```python
from build123d import *

# Parameters (mm, degrees)
SKETCH1_W                = 100
SKETCH1_H                = 67.6
BOSS_EXTRUDE1_DEPTH      = 3
SKETCH3_W                = 4
SKETCH3_H                = 3
CUT_EXTRUDE1_DEPTH       = 10
LPATTERN1_COUNT          = 13
LPATTERN1_PITCH          = 8
SKETCH7_W                = 15
SKETCH7_H                = 45
CUT_EXTRUDE5_DEPTH       = 3
MIRROR1_COPY_1_SKETCH_W  = 4
MIRROR1_COPY_1_SKETCH_H  = 3
MIRROR1_COPY_1_DEPTH     = 10
MIRROR1_COPY_2_SKETCH_W  = 4
MIRROR1_COPY_2_SKETCH_H  = 3
MIRROR1_COPY_2_DEPTH     = 10
MIRROR1_COPY_3_SKETCH_W  = 4
MIRROR1_COPY_3_SKETCH_H  = 3
MIRROR1_COPY_3_DEPTH     = 10
MIRROR1_COPY_4_SKETCH_W  = 4
MIRROR1_COPY_4_SKETCH_H  = 3
MIRROR1_COPY_4_DEPTH     = 10
MIRROR1_COPY_5_SKETCH_W  = 4
MIRROR1_COPY_5_SKETCH_H  = 3
MIRROR1_COPY_5_DEPTH     = 10
MIRROR1_COPY_6_SKETCH_W  = 4
MIRROR1_COPY_6_SKETCH_H  = 3
MIRROR1_COPY_6_DEPTH     = 10
MIRROR1_COPY_7_SKETCH_W  = 4
MIRROR1_COPY_7_SKETCH_H  = 3
MIRROR1_COPY_7_DEPTH     = 10
MIRROR1_COPY_8_SKETCH_W  = 4
MIRROR1_COPY_8_SKETCH_H  = 3
MIRROR1_COPY_8_DEPTH     = 10
MIRROR1_COPY_9_SKETCH_W  = 4
MIRROR1_COPY_9_SKETCH_H  = 3
MIRROR1_COPY_9_DEPTH     = 10
MIRROR1_COPY_10_SKETCH_W = 4
MIRROR1_COPY_10_SKETCH_H = 3
MIRROR1_COPY_10_DEPTH    = 10
MIRROR1_COPY_11_SKETCH_W = 4
MIRROR1_COPY_11_SKETCH_H = 3
MIRROR1_COPY_11_DEPTH    = 10
MIRROR1_COPY_12_SKETCH_W = 4
MIRROR1_COPY_12_SKETCH_H = 3
MIRROR1_COPY_12_DEPTH    = 10
LPATTERN2_COUNT          = 2
LPATTERN2_PITCH          = 30
LPATTERN2_COL_COUNT      = 2
LPATTERN2_COL_PITCH      = 30
SKETCH8_W                = 4
SKETCH8_H                = 8.2
SKETCH8_H_2              = 33.8
BOSS_EXTRUDE2_DEPTH      = 3
CUT_EXTRUDE6_REACH       = 5
SKETCH9_W                = 12
SKETCH9_H                = 3


with BuildPart() as part:
    # Sketch1 → Boss-Extrude1 (new body)
    with BuildSketch(Plane.XY):
        Rectangle(SKETCH1_W, SKETCH1_H)
    extrude(amount=BOSS_EXTRUDE1_DEPTH)

    # Sketch3 → Cut-Extrude1 (cut)
    with BuildSketch(Plane(origin=(0, 0, 0), x_dir=(-1, 0, 0), z_dir=(0, 0, -1))):
        with Locations((-48, -32.3)):
            Rectangle(SKETCH3_W, SKETCH3_H)
    cut_extrude1 = extrude(amount=-CUT_EXTRUDE1_DEPTH, mode=Mode.SUBTRACT)

    # LPattern1: Cut-Extrude1 ×13
    with Locations(*[(-i * LPATTERN1_PITCH, 0, 0) for i in range(1, LPATTERN1_COUNT)]):
        add(cut_extrude1, mode=Mode.SUBTRACT)

    # Sketch7 → Cut-Extrude5 (cut)
    with BuildSketch(Plane(origin=(0, 0, 0), x_dir=(-1, 0, 0), z_dir=(0, 0, -1))):
        Rectangle(SKETCH7_W, SKETCH7_H)
    cut_extrude5 = extrude(amount=-CUT_EXTRUDE5_DEPTH, mode=Mode.SUBTRACT)

    # Mirror1: Cut-Extrude1 across plane
    add(cut_extrude1.mirror(Plane.ZX), mode=Mode.SUBTRACT)

    # Mirror1 copy 1 sketch → Mirror1 copy 1 (cut)
    with BuildSketch(Plane(origin=(-8, 0, 0), x_dir=(-1, 0, 0), z_dir=(0, 0, -1))):
        with Locations((-48, 32.3)):
            Rectangle(MIRROR1_COPY_1_SKETCH_W, MIRROR1_COPY_1_SKETCH_H)
    extrude(amount=-MIRROR1_COPY_1_DEPTH, mode=Mode.SUBTRACT)

    # Mirror1 copy 2 sketch → Mirror1 copy 2 (cut)
    with BuildSketch(Plane(origin=(-16, 0, 0), x_dir=(-1, 0, 0), z_dir=(0, 0, -1))):
        with Locations((-48, 32.3)):
            Rectangle(MIRROR1_COPY_2_SKETCH_W, MIRROR1_COPY_2_SKETCH_H)
    extrude(amount=-MIRROR1_COPY_2_DEPTH, mode=Mode.SUBTRACT)

    # Mirror1 copy 3 sketch → Mirror1 copy 3 (cut)
    with BuildSketch(Plane(origin=(-24, 0, 0), x_dir=(-1, 0, 0), z_dir=(0, 0, -1))):
        with Locations((-48, 32.3)):
            Rectangle(MIRROR1_COPY_3_SKETCH_W, MIRROR1_COPY_3_SKETCH_H)
    extrude(amount=-MIRROR1_COPY_3_DEPTH, mode=Mode.SUBTRACT)

    # Mirror1 copy 4 sketch → Mirror1 copy 4 (cut)
    with BuildSketch(Plane(origin=(-32, 0, 0), x_dir=(-1, 0, 0), z_dir=(0, 0, -1))):
        with Locations((-48, 32.3)):
            Rectangle(MIRROR1_COPY_4_SKETCH_W, MIRROR1_COPY_4_SKETCH_H)
    extrude(amount=-MIRROR1_COPY_4_DEPTH, mode=Mode.SUBTRACT)

    # Mirror1 copy 5 sketch → Mirror1 copy 5 (cut)
    with BuildSketch(Plane(origin=(-40, 0, 0), x_dir=(-1, 0, 0), z_dir=(0, 0, -1))):
        with Locations((-48, 32.3)):
            Rectangle(MIRROR1_COPY_5_SKETCH_W, MIRROR1_COPY_5_SKETCH_H)
    extrude(amount=-MIRROR1_COPY_5_DEPTH, mode=Mode.SUBTRACT)

    # Mirror1 copy 6 sketch → Mirror1 copy 6 (cut)
    with BuildSketch(Plane(origin=(-48, 0, 0), x_dir=(-1, 0, 0), z_dir=(0, 0, -1))):
        with Locations((-48, 32.3)):
            Rectangle(MIRROR1_COPY_6_SKETCH_W, MIRROR1_COPY_6_SKETCH_H)
    extrude(amount=-MIRROR1_COPY_6_DEPTH, mode=Mode.SUBTRACT)

    # Mirror1 copy 7 sketch → Mirror1 copy 7 (cut)
    with BuildSketch(Plane(origin=(-56, 0, 0), x_dir=(-1, 0, 0), z_dir=(0, 0, -1))):
        with Locations((-48, 32.3)):
            Rectangle(MIRROR1_COPY_7_SKETCH_W, MIRROR1_COPY_7_SKETCH_H)
    extrude(amount=-MIRROR1_COPY_7_DEPTH, mode=Mode.SUBTRACT)

    # Mirror1 copy 8 sketch → Mirror1 copy 8 (cut)
    with BuildSketch(Plane(origin=(-64, 0, 0), x_dir=(-1, 0, 0), z_dir=(0, 0, -1))):
        with Locations((-48, 32.3)):
            Rectangle(MIRROR1_COPY_8_SKETCH_W, MIRROR1_COPY_8_SKETCH_H)
    extrude(amount=-MIRROR1_COPY_8_DEPTH, mode=Mode.SUBTRACT)

    # Mirror1 copy 9 sketch → Mirror1 copy 9 (cut)
    with BuildSketch(Plane(origin=(-72, 0, 0), x_dir=(-1, 0, 0), z_dir=(0, 0, -1))):
        with Locations((-48, 32.3)):
            Rectangle(MIRROR1_COPY_9_SKETCH_W, MIRROR1_COPY_9_SKETCH_H)
    extrude(amount=-MIRROR1_COPY_9_DEPTH, mode=Mode.SUBTRACT)

    # Mirror1 copy 10 sketch → Mirror1 copy 10 (cut)
    with BuildSketch(Plane(origin=(-80, 0, 0), x_dir=(-1, 0, 0), z_dir=(0, 0, -1))):
        with Locations((-48, 32.3)):
            Rectangle(MIRROR1_COPY_10_SKETCH_W, MIRROR1_COPY_10_SKETCH_H)
    extrude(amount=-MIRROR1_COPY_10_DEPTH, mode=Mode.SUBTRACT)

    # Mirror1 copy 11 sketch → Mirror1 copy 11 (cut)
    with BuildSketch(Plane(origin=(-88, 0, 0), x_dir=(-1, 0, 0), z_dir=(0, 0, -1))):
        with Locations((-48, 32.3)):
            Rectangle(MIRROR1_COPY_11_SKETCH_W, MIRROR1_COPY_11_SKETCH_H)
    extrude(amount=-MIRROR1_COPY_11_DEPTH, mode=Mode.SUBTRACT)

    # Mirror1 copy 12 sketch → Mirror1 copy 12 (cut)
    with BuildSketch(Plane(origin=(-96, 0, 0), x_dir=(-1, 0, 0), z_dir=(0, 0, -1))):
        with Locations((-48, 32.3)):
            Rectangle(MIRROR1_COPY_12_SKETCH_W, MIRROR1_COPY_12_SKETCH_H)
    extrude(amount=-MIRROR1_COPY_12_DEPTH, mode=Mode.SUBTRACT)

    # LPattern2: Cut-Extrude5 ×2
    with Locations(*[(-i * LPATTERN2_PITCH, 0, 0) for i in range(1, LPATTERN2_COUNT)]):
        add(cut_extrude5, mode=Mode.SUBTRACT)

    # LPattern2 col: Cut-Extrude5 ×2
    with Locations(*[(i * LPATTERN2_COL_PITCH, 0, 0) for i in range(1, LPATTERN2_COL_COUNT)]):
        add(cut_extrude5, mode=Mode.SUBTRACT)

    # Sketch8 → Boss-Extrude2 (add)
    with BuildSketch(Plane.XY.offset(3)):
        with Locations((24.5, -18.4)):
            Rectangle(SKETCH8_W, SKETCH8_H)
        with Locations((24.5, 5.6)):
            Rectangle(SKETCH8_W, SKETCH8_H_2)
        with Locations((35.5, 5.6)):
            Rectangle(SKETCH8_W, SKETCH8_H_2)
        with Locations((35.5, -18.4)):
            Rectangle(SKETCH8_W, SKETCH8_H)
    boss_extrude2 = extrude(amount=-BOSS_EXTRUDE2_DEPTH)

    # Mirror2: Boss-Extrude2 across plane
    add(boss_extrude2.mirror(Plane(origin=(0, 0, 0), x_dir=(0, 0, 1), z_dir=(1, 0, 0))))

    # Sketch9 → Cut-Extrude6 (cut, up to next)
    with BuildSketch(Plane(origin=(0, 0, 0), x_dir=(-1, 0, 0), z_dir=(0, 0, -1)), mode=Mode.PRIVATE) as cut_extrude6_sk1:
        with Locations((-44, 32.3)):
            Rectangle(SKETCH9_W, SKETCH9_H)
    cut_extrude6_tool1 = extrude(cut_extrude6_sk1.sketch, amount=-CUT_EXTRUDE6_REACH, mode=Mode.PRIVATE) & part.part
    add(cut_extrude6_tool1.solids().sort_by_distance((44, 32.3, 0))[0], mode=Mode.SUBTRACT)
    # Sketch9 → Cut-Extrude6 (cut, up to next)
    with BuildSketch(Plane(origin=(0, 0, 0), x_dir=(-1, 0, 0), z_dir=(0, 0, -1)), mode=Mode.PRIVATE) as cut_extrude6_sk2:
        with Locations((44, 32.3)):
            Rectangle(SKETCH9_W, SKETCH9_H)
    cut_extrude6_tool2 = extrude(cut_extrude6_sk2.sketch, amount=-CUT_EXTRUDE6_REACH, mode=Mode.PRIVATE) & part.part
    add(cut_extrude6_tool2.solids().sort_by_distance((-44, 32.3, 0))[0], mode=Mode.SUBTRACT)
    # Sketch9 → Cut-Extrude6 (cut, up to next)
    with BuildSketch(Plane(origin=(0, 0, 0), x_dir=(-1, 0, 0), z_dir=(0, 0, -1)), mode=Mode.PRIVATE) as cut_extrude6_sk3:
        with Locations((44, -32.3)):
            Rectangle(SKETCH9_W, SKETCH9_H)
    cut_extrude6_tool3 = extrude(cut_extrude6_sk3.sketch, amount=-CUT_EXTRUDE6_REACH, mode=Mode.PRIVATE) & part.part
    add(cut_extrude6_tool3.solids().sort_by_distance((-44, -32.3, 0))[0], mode=Mode.SUBTRACT)
    # Sketch9 → Cut-Extrude6 (cut, up to next)
    with BuildSketch(Plane(origin=(0, 0, 0), x_dir=(-1, 0, 0), z_dir=(0, 0, -1)), mode=Mode.PRIVATE) as cut_extrude6_sk4:
        with Locations((-44, -32.3)):
            Rectangle(SKETCH9_W, SKETCH9_H)
    cut_extrude6_tool4 = extrude(cut_extrude6_sk4.sketch, amount=-CUT_EXTRUDE6_REACH, mode=Mode.PRIVATE) & part.part
    add(cut_extrude6_tool4.solids().sort_by_distance((44, -32.3, 0))[0], mode=Mode.SUBTRACT)


solid = part.part
```
For this review, take the finished solid that the model builds, in its own axes (mm). A direction names the side the tool comes from. Give positions to 0.01 mm unless a question says otherwise; leave off trailing zeros. Write each loop counter-clockwise with the first axis right and the second up, starting at its lowest first coordinate (ties: lowest second). Pieces come first, ordered by that corner, then holes. Notation, with made-up numbers: M -21,29 L 32,29 A32 cw 32,59 Z; hole C -9.5,10.5 d11. An arc over 180 degrees is marked long. Answer as a JSON object with one key per item and string values. Group by question number.
Item 1: Tool access review of faces 3 (the flat face through (-30, 22.5, 1)), 4 (the flat face through (22, -32, 1)), 5 (the flat face through (-44, -30.8, 1)): name each direction out of +Z, -Z, +X, -X, +Y, -Y from which nothing blocks a thin tool from reaching the whole face with its end or side.
Item 2: Consider section B-B on z = 2.35. Count the separate pieces of the cut face and the enclosed holes in it, plus the area to 3 significant figures.
Item 3: Consider section C-C on x = 40.5. Write out the cut boundary in (y, z).
Item 4: Consider section A-A on y = -0.5. Write out the cut boundary in (x, z), plus the area to 3 significant figures.
Item 5: Draft analysis for pull direction X (two halves, no side actions). For faces 1 (the flat face through (-18, -32, 1)), 2 (the flat face through (-36, -33.8, 1)), state which applies: +X half, -X half, draft (parallel to the pull), parting line (faces both ways), or undercut.
Item 6: For probe 1 along X at (y, z) = (-20, 0.85); probe 2 along Y at (x, z) = (-23.5, 1.8); probe 3 along Y at (x, z) = (28.5, 2.7), list the stretches that pass through material, from the lowest coordinate up. Write a range as [from, to].
Item 7: For pin 1 Ø1.5 at (x, z) = (-23.5, 1) entering from -Y; pin 2 Ø0.9 at (y, z) = (33, 1) entering from -X; pin 3 Ø1.5 at (y, z) = (32, 2) entering from +X, all flat-tipped, find the tip position at first contact; note any pin that passes through.
Check result:
{
 "1": {"face 3": "+Z, -Z", "face 4": "+Z, -Z, -Y", "face 5": "+Z, -Z, -X, -Y"},
 "2": {"separate pieces": "1", "enclosed holes": "3", "area": "5,050 mm^2"},
 "3": {"outline": "M -30.8,0 L 30.8,0 L 30.8,3 L -30.8,3 Z"},
 "4": {"outline": "M -50,0 L -33.5,0 L -33.5,3 L -50,3 Z; M -26.5,0 L -7.5,0 L -7.5,3 L -26.5,3 Z; M 7.5,0 L 26.5,0 L 26.5,3 L 7.5,3 Z; M 33.5,0 L 50,0 L 50,3 L 33.5,3 Z", "area": "213 mm^2"},
 "5": {"face 1": "undercut", "face 2": "draft"},
 "6": {"probe 1": "x = [-50, -33.5], [-26.5, -7.5], [7.5, 26.5], [33.5, 50]", "probe 2": "y = [-30.8, -14.3], [-11.3, 30.8]", "probe 3": "y = [-33.8, -22.5], [22.5, 33.8]"},
 "7": {"pin 1": "stops at y = -30.8", "pin 2": "stops at x = -38", "pin 3": "stops at x = 38"}
}
